Verification items for the finished model (mm, model axes). Face numbers are marked on the shaded views. A direction names the side the tool comes from. Give positions to 0.01 mm unless a question says otherwise; leave off trailing zeros. Loops run counter-clockwise (first coordinate to the right, second up) from the corner with the lowest first, then second, coordinate; pieces in that order, holes last. Notation, with made-up numbers: (48, -23) - (104, -23) arc R16 ccw to (104, 0) - close; hole circle Ø7 at (-14.75, 85.5). An arc over 180 degrees is marked (long way). Answer in a Markdown table with one row per item.
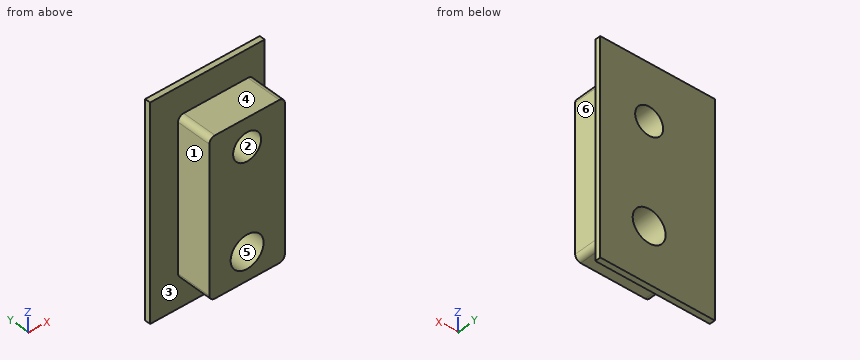
```python
from build123d import *

# Parameters (mm, degrees)
SKETCH1_W             = 6.75
SKETCH1_H             = 3.175
EXTRUDE1_DEPTH        = 7
SKETCH6_W             = 11.75
SKETCH6_H             = 19
EXTRUDE2_DEPTH        = 0.5
F_4_CLEARANCE_HOLE1_D = 2.9464
SKETCH3_R             = 1.25
CUT_EXTRUDE1_DEPTH    = 4.675
FILLET1_R             = 0.5
SKETCH16_W            = 19
SKETCH16_H            = 0.5
CUT_EXTRUDE7_DEPTH    = 1.5


with BuildPart() as part:
    # Sketch1 → Extrude1 (new body, symmetric)
    with BuildSketch(Plane.XY):
        with Locations((0, 115.5875)):
            Rectangle(SKETCH1_W, SKETCH1_H)
    extrude(amount=EXTRUDE1_DEPTH, both=True)

    # Sketch6 → Extrude2 (add)
    with BuildSketch(Plane(origin=(0, 117.175, 0), x_dir=(1, 0, 0), z_dir=(0, 1, 0))):
        Rectangle(SKETCH6_W, SKETCH6_H)
    extrude(amount=EXTRUDE2_DEPTH)

    # 4 Clearance Hole1 (through all)
    with Locations(Plane(origin=(-0.355703292, 117.675, 3.885176073), x_dir=(-1, 0, 0), z_dir=(0, 1, 0))):
        with Locations((-0.355703292, -8.385176073)):
            Hole(F_4_CLEARANCE_HOLE1_D / 2)

    # Sketch3 → Cut-Extrude1 (cut, through all)
    with BuildSketch(Plane(origin=(0, 117.675, 0), x_dir=(1, 0, 0), z_dir=(0, 1, 0))):
        with Locations(Location((0, -4.5, 0), (0, 0, 270))):  # turned: the seam where the file's is
            Circle(SKETCH3_R)
    extrude(amount=-CUT_EXTRUDE1_DEPTH, mode=Mode.SUBTRACT)

    # Fillet1
    fillet1_edges = [part.edges().sort_by_distance(p)[0] for p in [
        (-3.375, 115.5875, 7),
        (-3.375, 115.5875, -7),
        (3.375, 115.5875, -7),
        (3.375, 115.5875, 7),
    ]]
    fillet(fillet1_edges, radius=FILLET1_R)

    # Sketch16 → Cut-Extrude7 (cut)
    with BuildSketch(Plane(origin=(5.875, 0, 0), x_dir=(0, 0, -1), z_dir=(1, 0, 0))):
        with Locations((0, 117.425)):
            Rectangle(SKETCH16_W, SKETCH16_H)
    extrude(amount=-CUT_EXTRUDE7_DEPTH, mode=Mode.SUBTRACT)


solid = part.part
```
Q1. Sectioned sample at C-C (y = 116.45). Record the cut outline in (x, z) (3 decimals).
Completed:
| item | result |
|---|---|
| outline | (-3.375, -6.5) arc R0.5 ccw to (-2.875, -7) - (2.875, -7) arc R0.5 ccw to (3.375, -6.5) - (3.375, 6.5) arc R0.5 ccw to (2.875, 7) - (-2.875, 7) arc R0.5 ccw to (-3.375, 6.5) - close; hole circle Ø2.946 at (0, -4.5); hole circle Ø2.5 at (0, 4.5) |
Q2. Draft check along X on the marked faces 4, 5 and 6. Enter one of: +X half, -X half, draft (parallel to the pull), parting line (faces both ways), or undercut.
Completed:
| item | result |
|---|---|
| face 4 | draft |
| face 5 | undercut |
| face 6 | +X half |
Q3. Thickness scan on line 1 (X direction, y = 116.2, z = 4.5) (3 decimals); line 2 (Z direction, x = -0.75, y = 114.45); line 3 (X direction, y = 117.1, z = 0) (3 decimals). Record the ranges inside material, lowest first.
Completed:
| item | result |
|---|---|
| line 1 | -3.375 to -1.25, 1.25 to 3.375 |
| line 2 | -7 to -5.77, -3.23 to 3.5, 5.5 to 7 |
| line 3 | -3.375 to 3.375 |
Q4. Sectioned sample at B-B (x = 0). Record the cut outline in (y, z) (3 decimals), and give its area (3 significant figures).
Completed:
| item | result |
|---|---|
| outline | (114, -7) - (117.175, -7) - (117.175, -9.5) - (117.675, -9.5) - (117.675, -5.973) - (114, -5.973) - close; (114, -3.027) - (117.675, -3.027) - (117.675, 3.25) - (114, 3.25) - close; (114, 5.75) - (117.675, 5.75) - (117.675, 9.5) - (117.175, 9.5) - (117.175, 7) - (114, 7) - close |
| area | 33.9 mm^2 |
Q5. Go/stop test with flat-tipped pins: P1, Ø1.6, axis at x = -0.5, y = 115, coming from the -Z side; P2, Ø1.8, axis at x = 0, z = -4.5, coming from the -Y side. Record where each tip stops, or that it passes through.
Completed:
| item | result |
|---|---|
| P1 | z = -7 |
| P2 | through |
Q6. Tool access check on the marked faces 1, 2 and 3. Record the directions out of +Z, -Z, +X, -X, +Y, -Y that give a thin tool (end or side, any length) a straight path to the whole face; none if there is none.
Completed:
| item | result |
|---|---|
| face 1 | +Z, -Z, -X, -Y |
| face 2 | +Y, -Y |
| face 3 | -Y |
Q7. Sectioned sample at D-D (x = -2.25). Record the cut outline in (y, z) (3 decimals).
Completed:
| item | result |
|---|---|
| outline | (114, -7) - (117.175, -7) - (117.175, -9.5) - (117.675, -9.5) - (117.675, 9.5) - (117.175, 9.5) - (117.175, 7) - (114, 7) - close |
Q8. Sectioned sample at A-A (z = 4.5). Record the cut outline in (x, y) (3 decimals), and give its area (3 significant figures).
Completed:
| item | result |
|---|---|
| outline | (-5.875, 117.175) - (-3.375, 117.175) - (-3.375, 114) - (-1.25, 114) - (-1.25, 117.675) - (-5.875, 117.675) - close; (1.25, 114) - (3.375, 114) - (3.375, 117.175) - (4.375, 117.175) - (4.375, 117.675) - (1.25, 117.675) - close |
| area | 17.4 mm^2 |
